Here's how the part is built. I have some questions about the finished solid (model axes, mm). Face numbers are marked on the shaded views. A direction names the side the tool comes from. Give positions to 0.01 mm unless a question says otherwise; leave off trailing zeros. Write each loop counter-clockwise with the first axis right and the second up, starting at its lowest first coordinate (ties: lowest second). Pieces come first, ordered by that corner, then holes. Notation, with made-up numbers: (59, 6) -> (102, 6) arc R28 cw to (102, 24) -> close; hole circle Ø7 at (13, 32). An arc over 180 degrees is marked (long way). Return JSON: item names as keys, results as strings.
Autodesk Inventor part; units mm, degrees
ref_plane "Plano de trabajo1" through (0, 0, -15) normal (0, 0, 1) x (1, 0, 0)
ref_plane "YZ Plane" through (0, 0, 0) normal (1, 0, 0) x (0, 1, 0)
ref_plane "XZ Plane" through (0, 0, 0) normal (0, 1, 0) x (-1, 0, 0)
sketch "Boceto1" plane through (0, 0, 0) normal (0, 1, 0) x (-1, 0, 0)
  line L0 (0, 0) -> (-44, 0)
  line L1 (-44, 0) -> (-44, -30)
  line L2 (-44, -30) -> (0, -30)
  line L3 (0, -30) -> (0, 0)
  dimension "d0" = 30
  dimension "d1" = 44
extrude "Extrusión1" add sketch "Boceto1" along normal blind 8
sketch "Boceto2" plane through (0, 8, 0) normal (0, 1, 0) x (1, 0, 0)
  line L0 (-5.2329, 15) -> (48.4559, 15)
  line L1 (3, 26.5) -> (7.4, 26.5)
  line L2 (10.4, 23.5) -> (10.4, 6.5)
  line L3 (7.4, 3.5) -> (3, 3.5)
  line L4 (0, 6.5) -> (0, 15)
  line L5 (0, 30) -> (0, 0)
  line L6 (0, 15) -> (0, 23.5)
  arc A0 (0, 6.5) -> (3, 3.5) centre (3, 6.5) ccw
  arc A1 (3, 26.5) -> (0, 23.5) centre (3, 23.5) ccw
  arc A2 (10.4, 23.5) -> (7.4, 26.5) centre (7.4, 23.5) ccw
  arc A3 (7.4, 3.5) -> (10.4, 6.5) centre (7.4, 6.5) ccw
  line L7 (10.4, 15) -> (25.3, 15)
  line L8 (25.3, 15) -> (25.3, 19.9)
  line L9 (25.3, 19.9) -> (10.4, 19.9)
  line L10 (10.4, 19.9) -> (10.4, 15)
  line L11 (10.4, 15) -> (25.3, 15)
  line L12 (25.3, 15) -> (25.3, 10.1)
  line L13 (25.3, 10.1) -> (10.4, 10.1)
  line L14 (10.4, 10.1) -> (10.4, 15)
  line L15 (17.85, -3.2018) -> (17.85, 35.6428)
  line L16 (32.7, 26.5) -> (28.3, 26.5)
  line L17 (25.3, 23.5) -> (25.3, 6.5)
  line L18 (28.3, 3.5) -> (32.7, 3.5)
  line L19 (35.7, 6.5) -> (35.7, 15)
  line L20 (35.7, 15) -> (35.7, 23.5)
  arc A4 (32.7, 3.5) -> (35.7, 6.5) centre (32.7, 6.5) ccw
  arc A5 (35.7, 23.5) -> (32.7, 26.5) centre (32.7, 23.5) ccw
  arc A6 (28.3, 26.5) -> (25.3, 23.5) centre (28.3, 23.5) ccw
  arc A7 (25.3, 6.5) -> (28.3, 3.5) centre (28.3, 6.5) ccw
  line L21 (25.3, 19.9) -> (25.3, 15)
  line L22 (25.3, 10.1) -> (25.3, 15)
  point P0 (0, 26.5)
  point P1 (10.4, 26.5)
  point P2 (0, 3.5)
  point P3 (40.9329, 15)
  point P4 (35.7, 26.5)
  point P5 (25.3, 26.5)
  point P6 (35.7, 3.5)
  dimension "d5" = 11.5
  dimension "d6" = 11.5
  dimension "d7" = 10.4
  dimension "d8" = 3
  dimension "d9" = 14.9
  dimension "d10" = 4.9
  dimension "d11" = 4.9
  dimension "d12" = 9.8
  dimension "d13" = 35.7
extrude "Extrusión2" add sketch "Boceto2" along normal blind 15.5
sketch "Boceto3" plane through (0, 23.5, 0) normal (0, 1, 0) x (1, 0, 0)
  circle A0 centre (6.2, 15) radius 5.5
  circle A1 centre (29.5, 15) radius 5.5
  line L0 (0, 23.5) -> (0, 6.5)
  line L1 (35.7, 6.5) -> (35.7, 23.5)
  line L2 (10.4, 10.1) -> (10.4, 6.5)
  line L3 (10.4, 10.1) -> (10.4, 11.4489)
  line L4 (10.4, 19.9) -> (25.3, 19.9)
  line L5 (10.4, 18.5511) -> (10.4, 19.9)
  line L6 (10.4, 10.1) -> (25.3, 10.1)
  line L7 (25.3, 11.4489) -> (25.3, 10.1)
  line L8 (25.3, 18.5511) -> (25.3, 19.9)
  line L9 (25.3, 19.9) -> (10.4, 19.9)
  point P0 (0, 0)
  dimension "d16" = 6.2
  dimension "d17" = 6.2
  dimension "d18" = 11
  dimension "d19" = 11
  dimension "d26" = 23.3
extrude "Extrusión3" cut sketch "Boceto3" against normal blind 6 contours A0 L5 L4 L8 A1 L7 L6 L3
sketch "Boceto4" plane through (0, 23.5, 0) normal (0, 1, 0) x (1, 0, 0)
  arc A0 (10.4, 11.4489) -> (10.4, 18.5511) centre (6.2, 15) ccw
  circle A1 centre (6.2, 15) radius 3.9
  arc A2 (25.3, 18.5511) -> (25.3, 11.4489) centre (29.5, 15) ccw
  circle A3 centre (29.5, 15) radius 3.9
  point P0 (0, 0)
  dimension "d22" = 7.8
  dimension "d23" = 7.8
extrude "Extrusión4" cut sketch "Boceto4" against normal blind 12.5
sketch "Boceto5" plane through (6.2, 11, -15) normal (0, 1, 0) x (1, 0, 0)
  circle A0 centre (0, 0) radius 3.9
  circle A1 centre (0, 0) radius 1.25
  circle A2 centre (23.3, 0) radius 3.9
  circle A3 centre (23.3, 0) radius 1.25
  point P0 (-6.2, -15)
  dimension "d27" = 2.5
  dimension "d28" = 2.5
extrude "Extrusión5" cut sketch "Boceto5" against normal blind 8 contours A1 | A3
ref_plane "Plano de trabajo1" through (0, 0, -15) normal (0, 0, 1) x (1, 0, 0)
sketch "Boceto6" plane through (0, 0, -15) normal (0, 0, 1) x (1, 0, 0)
  line L0 (0, 8) -> (44, 8)
  line L1 (35.7, 8) -> (35.7, 23.5)
  line L2 (44, 8) -> (35.7, 8)
  line L3 (35.7, 8) -> (35.7, 16.3)
  line L4 (35.7, 16.3) -> (44, 8)
  point P0 (0, 0)
  dimension "d32" = 8.3
extrude "Extrusión6" add sketch "Boceto6" along normal mid plane 10
sketch "Boceto7" plane through (0, 0, 0) normal (0, -1, 0) x (1, 0, 0)
  line L0 (44, 0) -> (44, -30)
  line L1 (0, 0) -> (44, 0)
  line L2 (44, 0) -> (44, -30)
  line L3 (44, -30) -> (0, -30)
  line L4 (0, -30) -> (0, 0)
extrude "Extrusión7" cut sketch "Boceto7" against normal blind 8
properties part number "Primer inserto" material "Plastico PETG"
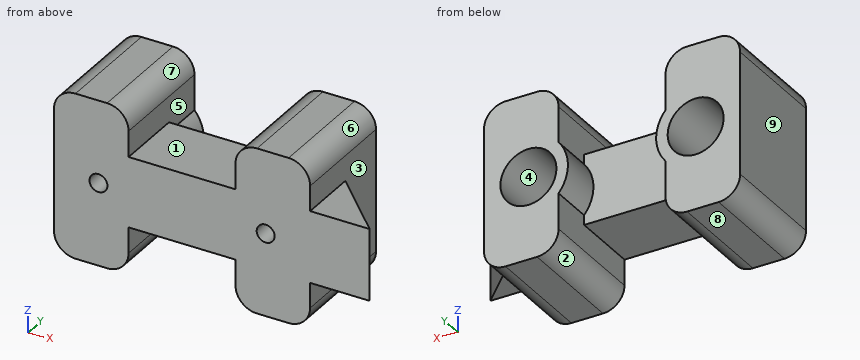
1. Suppose I cut it at A-A, the plane z = -15. List the corners of the cut face in (x, y) for me.
Taken from the geometry:
{"outline": "(0, 8) -> (4.95, 8) -> (4.95, 11) -> (2.3, 11) -> (2.3, 23.5) -> (0, 23.5) -> close; (7.45, 8) -> (28.25, 8) -> (28.25, 11) -> (25.6, 11) -> (25.6, 23.5) -> (24, 23.5) -> (24, 17.5) -> (11.7, 17.5) -> (11.7, 23.5) -> (10.1, 23.5) -> (10.1, 11) -> (7.45, 11) -> close; (30.75, 8) -> (44, 8) -> (35.7, 16.3) -> (35.7, 23.5) -> (33.4, 23.5) -> (33.4, 11) -> (30.75, 11) -> close"}
2. Which directions (+Z, -Z, +X, -X, +Y, -Y) give clear straight access to the entire face, cutting with the end or side of a thin tool? Please do the marked faces 1, 2, 3, 4 and 5.
Taken from the geometry:
{"face 1": "+Z, +Y, -Y", "face 2": "-Z, +Y, -Y", "face 3": "+X, +Y", "face 4": "+Y", "face 5": "+Z, +Y"}
3. For pin 1 Ø7.5 at (x, y) = (21.5, 13) entering from +Z; pin 2 Ø1.5 at (x, z) = (19.5, -18) entering from +Y; pin 3 Ø6.5 at (x, y) = (41, 12) entering from -Z, each with a flat end and sliding along its axis, tell me the tip position at first contact or that it passes through.
Taken from the geometry:
{"pin 1": "stops at z = -10.1", "pin 2": "stops at y = 17.5", "pin 3": "stops at z = -20"}
4. Suppose I cut it at D-D, the plane z = -20.75. List the corners of the cut face in (x, y) for me.
Taken from the geometry:
{"outline": "(0, 8) -> (10.4, 8) -> (10.4, 23.5) -> (0, 23.5) -> close; (25.3, 8) -> (35.7, 8) -> (35.7, 23.5) -> (25.3, 23.5) -> close"}
5. If I drill on line 1 (X direction, y = 22.75, z = -15); line 2 (X direction, y = 18, z = -20.5); line 3 (Z direction, x = 29.5, y = 10.2), over which ranges is the centre line in solid material (lowest first)? Write a range as [from, to].
Taken from the geometry:
{"line 1": "x = [0, 2.3], [10.1, 11.7], [24, 25.6], [33.4, 35.7]", "line 2": "x = [0, 10.4], [25.3, 35.7]", "line 3": "z = [-26.5, -16.25], [-13.75, -3.5]"}
6. If we mould it in two halves opening along X, with no side actions, what happens to the marked faces 6, 7, 8 and 9? For each: released by +X, released by -X, zero draft, split by the parting line, or undercut.
Taken from the geometry:
{"face 6": "released by +X", "face 7": "undercut", "face 8": "zero draft", "face 9": "released by -X"}
7. Suppose I cut it at B-B, the plane y = 15.75. List the corners of the cut face in (x, z) for me.
Taken from the geometry:
{"outline": "(0, -23.5) arc R3 ccw to (3, -26.5) -> (7.4, -26.5) arc R3 ccw to (10.4, -23.5) -> (10.4, -19.9) -> (25.3, -19.9) -> (25.3, -23.5) arc R3 ccw to (28.3, -26.5) -> (32.7, -26.5) arc R3 ccw to (35.7, -23.5) -> (35.7, -20) -> (36.25, -20) -> (36.25, -10) -> (35.7, -10) -> (35.7, -6.5) arc R3 ccw to (32.7, -3.5) -> (28.3, -3.5) arc R3 ccw to (25.3, -6.5) -> (25.3, -10.1) -> (10.4, -10.1) -> (10.4, -6.5) arc R3 ccw to (7.4, -3.5) -> (3, -3.5) arc R3 ccw to (0, -6.5) -> close; hole circle Ø7.8 at (6.2, -15); hole circle Ø7.8 at (29.5, -15)"}
8. Suppose I cut it at C-C, the plane x = 29.5. List the corners of the cut face in (y, z) for me.
Taken from the geometry:
{"outline": "(8, -26.5) -> (23.5, -26.5) -> (23.5, -18.9) -> (11, -18.9) -> (11, -16.25) -> (8, -16.25) -> close; (8, -13.75) -> (11, -13.75) -> (11, -11.1) -> (23.5, -11.1) -> (23.5, -3.5) -> (8, -3.5) -> close"}
